The figure shows three views and two pictorial views of one solid part (mm, origin at its lowest corner). Answer the questions. Coordinates: 2 decimals unless noted, no trailing zeros. Write each loop counter-clockwise with the first axis right and the second up, starting at its lowest first coordinate (ties: lowest second). Pieces come first, ordered by that corner, then holes.
Item 1: Section D-D (y = 4) is taken. Give the vertices of the cut face in (x, z).
Item 2: Section A-A (x = 46.5) is taken. Give the vertices of the cut face in (y, z), then the cut area to 3 significant figures.
Item 3: Section B-B (x = 25.75) is taken. Give the vertices of the cut face in (y, z), then the cut area to 3 significant figures.
Item 4: Determine the mould class of the marked faces 1, 2 and 3 for opening direction Z: released by +Z, released by -Z, zero draft, split by the parting line, or undercut.
Item 5: Straight lines are drawn through the part: probe 1 along X at (y, z) = (6.5, 46.5); probe 2 along X at (y, z) = (8.5, 19.5); probe 3 along Z at (x, y) = (67.25, 5.5). For each, find the intervals that lie inside material, in ascending order.
Item 6: Each of these flat-tipped pins is pushed along its axis until it touches: P1, Ø5, axis at y = 4.5, z = 40.5, coming from the -X side; P2, Ø2, axis at x = 67.25, z = 82.44, coming from the -Y side. Where does it stop, or does it pass through?
Item 7: Section C-C (z = 87) is taken. Give the vertices of the cut face in (x, y) (3 decimals).
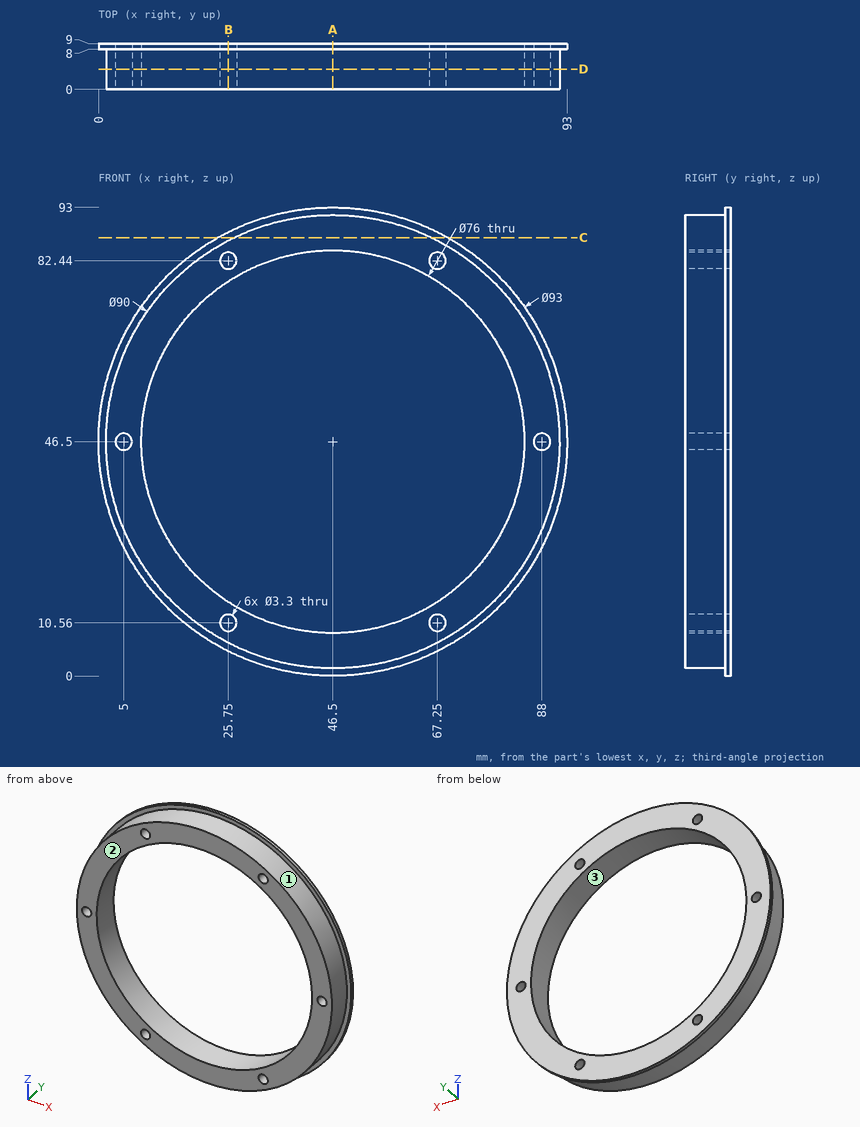
Established:
1. outline: circle Ø90 at (46.5, 46.5); hole circle Ø3.3 at (5, 46.5); hole circle Ø76 at (46.5, 46.5); hole circle Ø3.3 at (25.75, 10.56); hole circle Ø3.3 at (25.75, 82.44); hole circle Ø3.3 at (67.25, 10.56); hole circle Ø3.3 at (67.25, 82.44); hole circle Ø3.3 at (88, 46.5)
2. outline: (0, 1.5) - (8, 1.5) - (8, 0) - (9, 0) - (9, 8.5) - (0, 8.5) - close; (0, 84.5) - (9, 84.5) - (9, 93) - (8, 93) - (8, 91.5) - (0, 91.5) - close
2. area: 129 mm2
3. outline: (0, 6.57) - (8, 6.57) - (8, 4.89) - (9, 4.89) - (9, 8.91) - (0, 8.91) - close; (0, 12.21) - (9, 12.21) - (9, 14.67) - (0, 14.67) - close; (0, 78.33) - (9, 78.33) - (9, 80.79) - (0, 80.79) - close; (0, 84.09) - (9, 84.09) - (9, 88.11) - (8, 88.11) - (8, 86.43) - (0, 86.43) - close
3. area: 89.7 mm2
4. face 1: split by the parting line
4. face 2: zero draft
4. face 3: undercut
5. probe 1: x = 1.5 to 3.35, 6.65 to 8.5, 84.5 to 86.35, 89.65 to 91.5
5. probe 2: x = 8.64 to 19.76, 73.24 to 84.36
5. probe 3: z = 6.57 to 8.91, 12.21 to 14.67, 78.33 to 80.79, 84.09 to 86.43
6. P1: stops at x = 1.64
6. P2: passes through
7. outline: (23.653, 8) - (26.885, 8) - (26.885, 0) - (66.115, 0) - (66.115, 8) - (69.347, 8) - (69.347, 9) - (23.653, 9) - close
